Verification items for the finished model (mm, model axes). A direction names the side the tool comes from. Coordinates: 2 decimals unless noted, no trailing zeros. Order: outer loops, then holes, each group sorted by start corner. A loop starts at its lowest first (then second) coordinate and runs counter-clockwise, first axis right, second up.
Q1. Set-up check for faces 1 (the flat face through (19, 779, 0)), 2 (the flat face through (0, 801, -16.5)): record each of +Z, -Z, +X, -X, +Y, -Y from which the full face is reachable in a straight line by a thin tool's end or side.
Q2. Cross-section at B-B, the plane z = 9. Record the boundary of the cut face in (x, y), and give its area (3 significant figures).
Q3. Cross-section at C-C, the plane y = 1127.5. Record the boundary of the cut face in (x, z).
Q4. Draft check along Z on faces 3 (the flat face through (0, 801, 19)), 4 (the flat face through (0, 801, 16.5)), 5 (the flat face through (0, 19, -17)). Enter one of: pulls with the +Z half, pulls with the -Z half, needs draft (parallel to the pull), parting line crosses it, or undercut.
Q5. Cross-section at A-A, the plane x = 2.5. Record the boundary of the cut face in (y, z).
Q6. Thickness scan on line 1 (Z direction, x = -13, y = 881); line 2 (Y direction, x = 17, z = -1). Record the ranges inside material, lowest first.
from build123d import *

# Parameters (mm, degrees)
SALIENTE_EXTRUIR1_DEPTH = 2.5
SALIENTE_EXTRUIR2_DEPTH = 33
SALIENTE_EXTRUIR3_DEPTH = 33
SALIENTE_EXTRUIR4_DEPTH = 2.5


with BuildPart() as part:
    # Croquis1 → Saliente-Extruir1 (new body)
    with BuildSketch(Plane.XY.offset(19)):
        Polygon((19, 1542), (-19, 1580), (-19, 0), (19, 38), align=None)
    extrude(amount=-SALIENTE_EXTRUIR1_DEPTH)

    # Croquis2 → Saliente-Extruir2 (add)
    with BuildSketch(Plane(origin=(0, 0, 16.5), x_dir=(-1, 0, 0), z_dir=(0, 0, -1))):
        Polygon((-16.5, 1544.5), (-16.5, 35.5), (-19, 38), (-19, 1542), align=None)
    extrude(amount=SALIENTE_EXTRUIR2_DEPTH)

    # Croquis3 → Saliente-Extruir3 (add)
    with BuildSketch(Plane(origin=(0, 0, 16.5), x_dir=(-1, 0, 0), z_dir=(0, 0, -1))):
        Polygon((16.5, 2.5), (16.5, 1577.5), (19, 1580), (19, 0), align=None)
    extrude(amount=SALIENTE_EXTRUIR3_DEPTH)

    # Croquis4 → Saliente-Extruir4 (add)
    with BuildSketch(Plane(origin=(0, 0, -16.5), x_dir=(-1, 0, 0), z_dir=(0, 0, -1))):
        Polygon((-19, 1542), (19, 1580), (19, 0), (-19, 38), align=None)
    extrude(amount=SALIENTE_EXTRUIR4_DEPTH)


solid = part.part
Check values:
1. face 1: +Z, -Z, +X, +Y, -Y
1. face 2: +Y, -Y
2. outline: (-19, 0) - (-16.5, 2.5) - (-16.5, 1577.5) - (-19, 1580) - close; (16.5, 35.5) - (19, 38) - (19, 1542) - (16.5, 1544.5) - close
2. area: 7,710 mm2
3. outline: (-19, -19) - (19, -19) - (19, 19) - (-19, 19) - close; hole (-16.5, -16.5) - (16.5, -16.5) - (16.5, 16.5) - (-16.5, 16.5) - close
4. face 3: pulls with the +Z half
4. face 4: undercut
4. face 5: needs draft
5. outline: (21.5, -19) - (1558.5, -19) - (1558.5, -16.5) - (21.5, -16.5) - close; (21.5, 16.5) - (1558.5, 16.5) - (1558.5, 19) - (21.5, 19) - close
6. line 1: z = -19 to -16.5, 16.5 to 19
6. line 2: y = 36 to 1544
